Part model, mm, in its own coordinate system. Face numbers are marked on the shaded views. A direction names the side the tool comes from. Round coordinates to 2 decimals unless told otherwise and drop trailing zeros. Loops run counter-clockwise (first coordinate to the right, second up) from the corner with the lowest first, then second, coordinate; pieces in that order, holes last. Notation, with made-up numbers: (43, 10) - (91, 10) arc R11 cw to (91, 30) - close; hole circle Ø5 at (36.5, -24). An arc over 180 degrees is marked (long way). Write each question's results on one line, items separated by ' | '. Start each with the question number.
(1) Flat gauge pins, fed straight in: P1, Ø15.5, axis at x = -3, z = -6.5, coming from the -Y side; P2, Ø1, axis at x = 9.5, z = -12.5, coming from the -Y side; P3, Ø7, axis at y = -60, z = 12, coming from the -X side. Where does each tip first touch, or does it go through?
(2) Tool access for the marked faces 4 and 5: list every direction of +Z, -Z, +X, -X, +Y, -Y with a clear straight run to the whole face (end or side of a thin tool).
(3) Cut at D-D, the plane z = -2. List the corners of the cut face in (x, y), then the cut area to 3 significant figures.
(4) Cut at B-B, the plane z = 12. List the corners of the cut face in (x, y).
(5) Mould opens along X. For the marked faces 1, 2 and 3 say: released by +X, released by -X, zero draft, split by the parting line, or undercut.
(6) Drill centre lines: L1, parallel to X at y = -54, z = -1; L2, parallel to Y at x = -7, z = 10; L3, parallel to Y at x = -13.8, z = 12. Where is each one in solid material? Low to high.
(7) Cut at C-C, the plane y = -35.5. List the corners of the cut face in (x, z), then the cut area to 3 significant figures.
(8) Cut at A-A, the plane x = 0. List the corners of the cut face in (y, z), then the cut area to 3 significant figures.
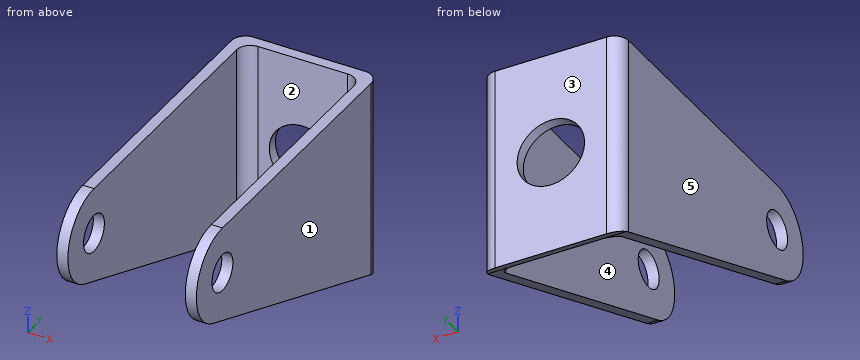
from build123d import *

# Parameters (mm, degrees)
CROQUIS1_W              = 30
CROQUIS1_H              = 44
CROQUIS1_R              = 7.25
SALIENTE_EXTRUIR1_DEPTH = 2.38
CROQUIS2_R              = 4
SALIENTE_EXTRUIR2_DEPTH = 2.38
CORTAR_EXTRUIR1_DEPTH   = 31
CROQUIS4_R              = 4
SALIENTE_EXTRUIR3_DEPTH = 2.38
REDONDEO1_R             = 3
REDONDEO2_R             = 3
REDONDEO3_R             = 3


with BuildPart() as part:
    # Croquis1 → Saliente-Extruir1 (new body)
    with BuildSketch(Plane(origin=(0, 0, 0), x_dir=(1, 0, 0), z_dir=(0, 1, 0))):
        Rectangle(CROQUIS1_W, CROQUIS1_H)
        Circle(CROQUIS1_R, mode=Mode.SUBTRACT)
    extrude(amount=-SALIENTE_EXTRUIR1_DEPTH)

    # Croquis2 → Saliente-Extruir2 (add)
    with BuildSketch(Plane(origin=(15, 0, 0), x_dir=(0, 0, -1), z_dir=(1, 0, 0))):
        with BuildLine():
            Line((-22, -60), (-22, 0))
            Line((-22, 0), (22, 0))
            Line((22, 0), (-2.676843343, -63.616455439))
            ThreePointArc((-2.676843343, -63.616455439), (-13.839624069, -69.8293328), (-22, -60))
        make_face()
        with Locations((-12, -60)):
            Circle(CROQUIS2_R, mode=Mode.SUBTRACT)
    extrude(amount=-SALIENTE_EXTRUIR2_DEPTH)

    # Croquis3 → Cortar-Extruir1 (cut, through all)
    with BuildSketch(Plane(origin=(15, 0, 0), x_dir=(0, 0, -1), z_dir=(1, 0, 0))):
        Polygon((22, 0), (21.076797241, -2.38), (22, -2.38), align=None)
    extrude(amount=-CORTAR_EXTRUIR1_DEPTH, mode=Mode.SUBTRACT)

    # Croquis4 → Saliente-Extruir3 (add)
    with BuildSketch(Plane.ZY.offset(15)):
        with BuildLine():
            Line((-22, 0), (2.676843343, -63.616455439))
            ThreePointArc((2.676843343, -63.616455439), (13.839624069, -69.8293328), (22, -60))
            Line((22, -60), (22, 0))
            Line((22, 0), (-22, 0))
        make_face()
        with Locations((12, -60)):
            Circle(CROQUIS4_R, mode=Mode.SUBTRACT)
    extrude(amount=-SALIENTE_EXTRUIR3_DEPTH)

    # Redondeo1
    redondeo1_edges = [part.edges().sort_by_distance(p)[0] for p in [
        (12.62, -2.38, 0.461601379),
    ]]
    fillet(redondeo1_edges, radius=REDONDEO1_R)

    # Redondeo2
    redondeo2_edges = [part.edges().sort_by_distance(p)[0] for p in [
        (-12.62, -2.38, 0.461601379),
    ]]
    fillet(redondeo2_edges, radius=REDONDEO2_R)

    # Redondeo3
    redondeo3_edges = [part.edges().sort_by_distance(p)[0] for p in [
        (-15, 0, 0),
        (15, 0, 0),
    ]]
    fillet(redondeo3_edges, radius=REDONDEO3_R)


solid = part.part
A:
1) P1: y = -2.6 | P2: y = -2.4 | P3: through
2) face 4: +Z, -Z, -Y | face 5: +Z, -Z, -X, +Y, -Y
3) outline: (-15, -51.56) - (-12.62, -51.56) - (-12.62, -5.38) arc R3 cw to (-9.62, -2.38) - (-6.97, -2.38) - (-6.97, 0) - (-12, 0) arc R3 ccw to (-15, -3) - close; (6.97, -2.38) - (9.62, -2.38) arc R3 cw to (12.62, -5.38) - (12.62, -51.56) - (15, -51.56) - (15, -3) arc R3 ccw to (12, 0) - (6.97, 0) - close | area: 272 mm2
4) outline: (-15, -70) - (-12.62, -70) - (-12.62, -64) - (-15, -64) - close; (-15, -56) - (-12.62, -56) - (-12.62, -5.38) arc R3 cw to (-9.62, -2.38) - (9.62, -2.38) arc R3 cw to (12.62, -5.38) - (12.62, -56) - (15, -56) - (15, -3) arc R3 ccw to (12, 0) - (-12, 0) arc R3 ccw to (-15, -3) - close; (12.62, -70) - (15, -70) - (15, -64) - (12.62, -64) - close
5) face 1: released by +X | face 2: undercut | face 3: zero draft
6) L1: -15 to -12.62, 12.62 to 15 | L2: -2.38 to 0 | L3: -70 to -64, -56 to -0.6
7) outline: (-15, -8.23) - (-12.62, -8.23) - (-12.62, 22) - (-15, 22) - close; (12.62, -8.23) - (15, -8.23) - (15, 22) - (12.62, 22) - close | area: 144 mm2
8) outline: (-2.38, -21.08) - (0, -22) - (0, -7.25) - (-2.38, -7.25) - close; (-2.38, 7.25) - (0, 7.25) - (0, 22) - (-2.38, 22) - close | area: 69.1 mm2
